from build123d import *

# Parameters (mm, degrees)
CUT_EXTRUDE1_DEPTH      = 15.558488421
CUT_EXTRUDE1_DEPTH_BACK = 15.558488421
SKETCH2_W               = 4.202041029
SKETCH2_H               = 2


with BuildPart() as part:
    # Sketch1 → Revolve1 (revolve)
    with BuildSketch(Plane(origin=(0, 0, 0), x_dir=(0, 0, -1), z_dir=(1, 0, 0)), mode=Mode.PRIVATE) as revolve1_sk:
        with BuildLine():
            Line((2.274058577, 0), (2.274058577, 2))
            Line((2.274058577, 2), (1.274058577, 2))
            Line((1.274058577, 2), (1.274058577, 3))
            Line((1.274058577, 3), (-5.725941423, 3))
            Line((-5.725941423, 3), (-5.725941423, 5))
            Line((-5.725941423, 5), (-7.725941423, 5))
            ThreePointArc((-7.725941423, 5), (-11.261475329, 3.535533906), (-12.725941423, 0))
            Line((-12.725941423, 0), (2.274058577, 0))
        make_face()
    revolve(revolve1_sk.sketch.rotate(Axis((0, 0, 24), (0, 0, -1)), 180), axis=Axis((0, 0, 24), (0, 0, -1)))

    # Sketch2 → Cut-Extrude1 (cut, two sides: drawn at the far end of the back side and taken through both)
    with BuildSketch(Plane(origin=(0, 0, 0), x_dir=(0, 0, -1), z_dir=(1, 0, 0)).offset(-CUT_EXTRUDE1_DEPTH_BACK)):
        with Locations((-12.725941423, 0)):
            Rectangle(SKETCH2_W, SKETCH2_H)
    extrude(amount=CUT_EXTRUDE1_DEPTH + CUT_EXTRUDE1_DEPTH_BACK, mode=Mode.SUBTRACT)


solid = part.part
Check sheet for the modelled part. Datum: model origin and axes. Units: mm. A direction names the side the tool comes from. Round coordinates to 2 decimals unless told otherwise and drop trailing zeros. Order: outer loops, then holes, each group sorted by start corner. A loop starts at its lowest first (then second) coordinate and runs counter-clockwise, first axis right, second up.
Q1. Scan lines: L1, parallel to Z at x = -3.5, y = 0.25; L2, parallel to X at y = -4, z = 6.5; L3, parallel to Z at x = -1.5, y = 0.5. Record each from-to range of solid material in increasing order.
Filled sheet:
L1: z = 5.73 to 10.62
L2: x = -3 to 3
L3: z = -2.27 to 10.62
Q2. Cross-section at D-D, the plane x = -3.5. Enter the section's corners in (y, z), plus the area to 3 significant figures.
Filled sheet:
outline: (-3.57, 5.73) - (3.57, 5.73) - (3.57, 7.73) arc R3.57 ccw to (1, 11.15) - (1, 10.62) - (-1, 10.62) - (-1, 11.15) arc R3.57 ccw to (-3.57, 7.73) - close
area: 33.1 mm2
Q3. Cross-section at A-A, the plane y = 0. Enter the section's corners in (x, z), plus the area to 3 significant figures.
Filled sheet:
outline: (-5, 5.73) - (-3, 5.73) - (-3, -1.27) - (-2, -1.27) - (-2, -2.27) - (2, -2.27) - (2, -1.27) - (3, -1.27) - (3, 5.73) - (5, 5.73) - (5, 7.73) arc R5 ccw to (4.07, 10.62) - (-4.07, 10.62) arc R5 ccw to (-5, 7.73) - close
area: 93.3 mm2
Q4. Draft check along Y on faces 1 (the face through (2, 0, -2)), 2 (the face through (3.3, -0.1, 5.726)), 3 (the face through (0, 0, 10.625)). Enter one of: pulls with the +Y half, pulls with the -Y half, needs draft (parallel to the pull), parting line crosses it, or undercut.
Filled sheet:
face 1: parting line crosses it
face 2: needs draft
face 3: undercut
Q5. Cross-section at C-C, the plane z = 0.75. Enter the section's corners in (x, y).
Filled sheet:
outline: circle Ø6 at (0, 0)
Q6. Depth check by flat-ended pin: P1, Ø1.5, axis at x = 2, z = 2.5, coming from the -Y side; P2, Ø2, axis at x = -0.5, z = 4, coming from the -Y side; P3, Ø5, axis at y = -4, z = 10.5, coming from the -X side. Enter the tip coordinate at first touch or a pass-through.
Filled sheet:
P1: stops at y = -2.73
P2: stops at y = -3
P3: stops at x = -4.4
Q7. Set-up check for faces 4 (the face through (-0.9, -2.86, 2.27)), 5 (the face through (0, 1, 11)), 6 (the face through (0, 5, 7)): record each of +Z, -Z, +X, -X, +Y, -Y from which the full face is reachable in a straight line by a thin tool's end or side.
Filled sheet:
face 4: -Z
face 5: +Z, +X, -X
face 6: +Z, -Z
Q8. Cross-section at B-B, the plane x = 0. Enter the section's corners in (y, z), plus the area to 3 significant figures.
Filled sheet:
outline: (-5, 5.73) - (-3, 5.73) - (-3, -1.27) - (-2, -1.27) - (-2, -2.27) - (2, -2.27) - (2, -1.27) - (3, -1.27) - (3, 5.73) - (5, 5.73) - (5, 7.73) arc R5 ccw to (1, 12.62) - (1, 10.62) - (-1, 10.62) - (-1, 12.62) arc R5 ccw to (-5, 7.73) - close
area: 101 mm2
